from build123d import *

# Parameters (mm, degrees)
SKETCH_1_R      = 2
SKETCH_1_R_2    = 1
EXTRUDE_1_DEPTH = 72
SKETCH_2_W      = 0.5
SKETCH_2_H      = 3
SKETCH_3_W      = 0.5
SKETCH_3_H      = 47


with BuildPart() as part:
    # Эскиз1 → Бобышка-Вытянуть1 (new body)
    with BuildSketch(Plane(origin=(0, 0, 0), x_dir=(1, 0, 0), z_dir=(0, 1, 0))):
        Circle(SKETCH_1_R)
        Circle(SKETCH_1_R_2, mode=Mode.SUBTRACT)
    extrude(amount=EXTRUDE_1_DEPTH)

    # Эскиз2 → Вырез-Повернуть1 (revolve, cut)
    with BuildSketch(Plane.XY):
        with Locations((1.75, 70.5)):
            Rectangle(SKETCH_2_W, SKETCH_2_H)
        with Locations((1.75, 63.5)):
            Rectangle(SKETCH_2_W, SKETCH_2_H)
    revolve(axis=Axis((0, 72, 0), (0, -1, 0)), mode=Mode.SUBTRACT)

    # Эскиз3 → Вырез-Повернуть2 (revolve, cut)
    with BuildSketch(Plane.XY):
        with Locations((1.75, 23.5)):
            Rectangle(SKETCH_3_W, SKETCH_3_H)
    revolve(axis=Axis((0, 0, 0), (0, 1, 0)), mode=Mode.SUBTRACT)


solid = part.part
Geometry check sheet. Reference: the model listing, model coordinates, mm. A direction names the side the tool comes from. Give positions to 0.01 mm unless a question says otherwise; leave off trailing zeros. Loops run counter-clockwise (first coordinate to the right, second up) from the corner with the lowest first, then second, coordinate; pieces in that order, holes last. Notation, with made-up numbers: M 24.25,78.5 L 57.25,78.5 A23 ccw 57.25,89.5 Z; hole C -14,53 d1. An arc over 180 degrees is marked long. Answer as a JSON object with one key per item and string values. Group by question number.
Item 1: Sectioned sample at B-B on x = 0. Record the boundary of the cut face in (y, z).
Item 2: Access from +Z, -Z, +X, -X, +Y, -Y to the whole of each face (thin tool, end or side, straight path). Record for faces 1 (the cylindrical face through (0, 67, 2)), 2 (the cylindrical face through (-1.5, 70.52, 0.07)), 3 (the cylindrical face through (-1.5, 23.83, -0.07)).
Item 3: Sectioned sample at D-D on y = 61. Record the boundary of the cut face in (x, z).
Item 4: Sectioned sample at A-A on z = 0. Record the boundary of the cut face in (x, y), plus the area to 3 significant figures.
Item 5: Sectioned sample at C-C on y = 9. Record the boundary of the cut face in (x, z).
Item 6: Material ranges on L1, parallel to X at y = 27, z = 0.05; L2, parallel to Z at x = 0, y = 57, recorded low to high.
Item 7: Mould release check, pull along Y, two halves, no side actions. Record for faces 4 (the cylindrical face through (-1.5, 63.52, 0.07)), 5 (the cylindrical face through (0, 54, 2)): pulls with the +Y half, pulls with the -Y half, needs draft (parallel to the pull), parting line crosses it, or undercut.
Findings below:
{
 "1": {"outline": "M 0,-1.5 L 47,-1.5 L 47,-2 L 62,-2 L 62,-1.5 L 65,-1.5 L 65,-2 L 69,-2 L 69,-1.5 L 72,-1.5 L 72,-1 L 0,-1 Z; M 0,1 L 72,1 L 72,1.5 L 69,1.5 L 69,2 L 65,2 L 65,1.5 L 62,1.5 L 62,2 L 47,2 L 47,1.5 L 0,1.5 Z"},
 "2": {"face 1": "+Y, -Y", "face 2": "+Y", "face 3": "-Y"},
 "3": {"outline": "C 0,0 d4; hole C 0,0 d2"},
 "4": {"outline": "M -2,47 L -1.5,47 L -1.5,0 L -1,0 L -1,72 L -1.5,72 L -1.5,69 L -2,69 L -2,65 L -1.5,65 L -1.5,62 L -2,62 Z; M 1,0 L 1.5,0 L 1.5,47 L 2,47 L 2,62 L 1.5,62 L 1.5,65 L 2,65 L 2,69 L 1.5,69 L 1.5,72 L 1,72 Z", "area": "91.0 mm2"},
 "5": {"outline": "C 0,0 d3; hole C 0,0 d2"},
 "6": {"L1": "-1.5 to -1, 1 to 1.5", "L2": "-2 to -1, 1 to 2"},
 "7": {"face 4": "undercut", "face 5": "needs draft"}
}
